from build123d import *

# Parameters (mm, degrees)
SKETCH1_W                  = 105
SKETCH1_H                  = 100
SKETCH1_W_2                = 4
SKETCH1_H_2                = 11
MAIN_PCB_DEPTH             = 1.25
MAIN_PCB_ROUNDED_CORNERS_R = 5
MAIN_PCB_HOLES_REACH       = 3.25
SKETCH2_R                  = 2
SKETCH2_R_2                = 1.375


with BuildPart() as part:
    # Sketch1 → Main PCB (new body)
    with BuildSketch(Plane(origin=(0, 0, 0), x_dir=(1, 0, 0), z_dir=(0, 1, 0))):
        Rectangle(SKETCH1_W, SKETCH1_H)
        with Locations((54.5, 19)):
            Rectangle(SKETCH1_W_2, SKETCH1_H_2)
    extrude(amount=MAIN_PCB_DEPTH)

    # Main PCB rounded corners
    main_pcb_rounded_corners_edges = [part.edges().sort_by_distance(p)[0] for p in [
        (52.5, 0.625, 50),
        (-52.5, 0.625, 50),
        (-52.5, 0.625, -50),
        (52.5, 0.625, -50),
    ]]
    fillet(main_pcb_rounded_corners_edges, radius=MAIN_PCB_ROUNDED_CORNERS_R)

    # Sketch2 → Main PCB holes (cut, up to next)
    with BuildSketch(Plane(origin=(0, 1.25, 0), x_dir=(1, 0, 0), z_dir=(0, 1, 0)), mode=Mode.PRIVATE) as main_pcb_holes_sk1:
        with Locations((-46.9, 46.65)):
            Circle(SKETCH2_R)
    main_pcb_holes_tool1 = extrude(main_pcb_holes_sk1.sketch, amount=-MAIN_PCB_HOLES_REACH, mode=Mode.PRIVATE) & part.part
    add(main_pcb_holes_tool1.solids().sort_by_distance((-46.9, 1.25, -46.65))[0], mode=Mode.SUBTRACT)
    # Sketch2 → Main PCB holes (cut, up to next)
    with BuildSketch(Plane(origin=(0, 1.25, 0), x_dir=(1, 0, 0), z_dir=(0, 1, 0)), mode=Mode.PRIVATE) as main_pcb_holes_sk2:
        with Locations((46.9, 46.65)):
            Circle(SKETCH2_R)
    main_pcb_holes_tool2 = extrude(main_pcb_holes_sk2.sketch, amount=-MAIN_PCB_HOLES_REACH, mode=Mode.PRIVATE) & part.part
    add(main_pcb_holes_tool2.solids().sort_by_distance((46.9, 1.25, -46.65))[0], mode=Mode.SUBTRACT)
    # Sketch2 → Main PCB holes (cut, up to next)
    with BuildSketch(Plane(origin=(0, 1.25, 0), x_dir=(1, 0, 0), z_dir=(0, 1, 0)), mode=Mode.PRIVATE) as main_pcb_holes_sk3:
        with Locations((46.9, -46.65)):
            Circle(SKETCH2_R)
    main_pcb_holes_tool3 = extrude(main_pcb_holes_sk3.sketch, amount=-MAIN_PCB_HOLES_REACH, mode=Mode.PRIVATE) & part.part
    add(main_pcb_holes_tool3.solids().sort_by_distance((46.9, 1.25, 46.65))[0], mode=Mode.SUBTRACT)
    # Sketch2 → Main PCB holes (cut, up to next)
    with BuildSketch(Plane(origin=(0, 1.25, 0), x_dir=(1, 0, 0), z_dir=(0, 1, 0)), mode=Mode.PRIVATE) as main_pcb_holes_sk4:
        with Locations((-46.9, -46.65)):
            Circle(SKETCH2_R)
    main_pcb_holes_tool4 = extrude(main_pcb_holes_sk4.sketch, amount=-MAIN_PCB_HOLES_REACH, mode=Mode.PRIVATE) & part.part
    add(main_pcb_holes_tool4.solids().sort_by_distance((-46.9, 1.25, 46.65))[0], mode=Mode.SUBTRACT)
    # Sketch2 → Main PCB holes (cut, up to next)
    with BuildSketch(Plane(origin=(0, 1.25, 0), x_dir=(1, 0, 0), z_dir=(0, 1, 0)), mode=Mode.PRIVATE) as main_pcb_holes_sk5:
        with Locations((-36.75, -48.625)):
            Circle(SKETCH2_R_2)
    main_pcb_holes_tool5 = extrude(main_pcb_holes_sk5.sketch, amount=-MAIN_PCB_HOLES_REACH, mode=Mode.PRIVATE) & part.part
    add(main_pcb_holes_tool5.solids().sort_by_distance((-36.75, 1.25, 48.625))[0], mode=Mode.SUBTRACT)
    # Sketch2 → Main PCB holes (cut, up to next)
    with BuildSketch(Plane(origin=(0, 1.25, 0), x_dir=(1, 0, 0), z_dir=(0, 1, 0)), mode=Mode.PRIVATE) as main_pcb_holes_sk6:
        with BuildLine():
            ThreePointArc((-36.75, -50), (-37.722271824, -49.597271824), (-38.125, -48.625))
            Line((-38.125, -48.625), (-38.125, -50))
            Line((-38.125, -50), (-36.75, -50))
        make_face()
    main_pcb_holes_tool6 = extrude(main_pcb_holes_sk6.sketch, amount=-MAIN_PCB_HOLES_REACH, mode=Mode.PRIVATE) & part.part
    add(main_pcb_holes_tool6.solids().sort_by_distance((-37.817869, 1.25, 49.692869))[0], mode=Mode.SUBTRACT)
    # Sketch2 → Main PCB holes (cut, up to next)
    with BuildSketch(Plane(origin=(0, 1.25, 0), x_dir=(1, 0, 0), z_dir=(0, 1, 0)), mode=Mode.PRIVATE) as main_pcb_holes_sk7:
        with BuildLine():
            Line((-35.375, -50), (-35.375, -48.625))
            ThreePointArc((-35.375, -48.625), (-35.777728176, -49.597271824), (-36.75, -50))
            Line((-36.75, -50), (-35.375, -50))
        make_face()
    main_pcb_holes_tool7 = extrude(main_pcb_holes_sk7.sketch, amount=-MAIN_PCB_HOLES_REACH, mode=Mode.PRIVATE) & part.part
    add(main_pcb_holes_tool7.solids().sort_by_distance((-35.682131, 1.25, 49.692869))[0], mode=Mode.SUBTRACT)
    # Sketch2 → Main PCB holes (cut, up to next)
    with BuildSketch(Plane(origin=(0, 1.25, 0), x_dir=(1, 0, 0), z_dir=(0, 1, 0)), mode=Mode.PRIVATE) as main_pcb_holes_sk8:
        with BuildLine():
            Line((-36.75, 50), (-38.125, 50))
            Line((-38.125, 50), (-38.125, 48.625))
            ThreePointArc((-38.125, 48.625), (-37.722271824, 49.597271824), (-36.75, 50))
        make_face()
    main_pcb_holes_tool8 = extrude(main_pcb_holes_sk8.sketch, amount=-MAIN_PCB_HOLES_REACH, mode=Mode.PRIVATE) & part.part
    add(main_pcb_holes_tool8.solids().sort_by_distance((-37.817869, 1.25, -49.692869))[0], mode=Mode.SUBTRACT)
    # Sketch2 → Main PCB holes (cut, up to next)
    with BuildSketch(Plane(origin=(0, 1.25, 0), x_dir=(1, 0, 0), z_dir=(0, 1, 0)), mode=Mode.PRIVATE) as main_pcb_holes_sk9:
        with Locations((-36.75, 48.625)):
            Circle(SKETCH2_R_2)
    main_pcb_holes_tool9 = extrude(main_pcb_holes_sk9.sketch, amount=-MAIN_PCB_HOLES_REACH, mode=Mode.PRIVATE) & part.part
    add(main_pcb_holes_tool9.solids().sort_by_distance((-36.75, 1.25, -48.625))[0], mode=Mode.SUBTRACT)
    # Sketch2 → Main PCB holes (cut, up to next)
    with BuildSketch(Plane(origin=(0, 1.25, 0), x_dir=(1, 0, 0), z_dir=(0, 1, 0)), mode=Mode.PRIVATE) as main_pcb_holes_sk10:
        with BuildLine():
            Line((-35.375, 50), (-36.75, 50))
            ThreePointArc((-36.75, 50), (-35.777728176, 49.597271824), (-35.375, 48.625))
            Line((-35.375, 48.625), (-35.375, 50))
        make_face()
    main_pcb_holes_tool10 = extrude(main_pcb_holes_sk10.sketch, amount=-MAIN_PCB_HOLES_REACH, mode=Mode.PRIVATE) & part.part
    add(main_pcb_holes_tool10.solids().sort_by_distance((-35.682131, 1.25, -49.692869))[0], mode=Mode.SUBTRACT)


solid = part.part
Model file for the job. Use its own axes, mm. Give positions to 0.01 mm unless a question says otherwise; leave off trailing zeros. Order: outer loops, then holes, each group sorted by start corner. A loop starts at its lowest first (then second) coordinate and runs counter-clockwise, first axis right, second up. Notation, with made-up numbers: (-27, -32.75) - (-19, -32.75) arc R25 cw to (-19, -6.75) - close; hole circle Ø3 at (38, 34). An arc over 180 degrees is marked (long way). One line per item, written item: value.
Item 1: Two-plate mould, pull along Z, no slides. Class faces 1 (the cylindrical face through (46.466, 0.634, 48.602)), 2 (the cylindrical face through (51, 0.63, 48.57)), 3 (the flat face through (1, 0, -1)): released by +Z, released by -Z, zero draft, split by the parting line, or undercut.
Response values:
face 1: undercut
face 2: released by +Z
face 3: zero draft
Item 2: Slice it at C-C (x = -36.75). List the corners of the cut face in (y, z).
Response values:
outline: (0, -47.25) - (1.25, -47.25) - (1.25, 47.25) - (0, 47.25) - close
Item 3: Slice it at A-A (y = 0.85). List the corners of the cut face in (x, z) (3 decimals).
Response values:
outline: (-52.5, -45) arc R5 ccw to (-47.5, -50) - (-38.125, -50) - (-38.125, -48.625) arc R1.375 cw to (-35.375, -48.625) - (-35.375, -50) - (47.5, -50) arc R5 ccw to (52.5, -45) - (52.5, -24.5) - (56.5, -24.5) - (56.5, -13.5) - (52.5, -13.5) - (52.5, 45) arc R5 ccw to (47.5, 50) - (-35.375, 50) - (-35.375, 48.625) arc R1.375 cw to (-38.125, 48.625) - (-38.125, 50) - (-47.5, 50) arc R5 ccw to (-52.5, 45) - close; hole circle Ø4 at (-46.9, -46.65); hole circle Ø4 at (-46.9, 46.65); hole circle Ø4 at (46.9, -46.65); hole circle Ø4 at (46.9, 46.65)
Item 4: Pin check, flat tips, straight feed: pin 1 Ø3 at (x, z) = (-46.9, -46.65) entering from +Y; pin 2 Ø0.6 at (y, z) = (0.5, 49.5) entering from +X. Stop position of each tip, or through.
Response values:
pin 1: through
pin 2: x = 50.21
Item 5: Slice it at B-B (z = 43). List the corners of the cut face in (x, y), then the cut area to 3 significant figures.
Response values:
outline: (-52.5, 0) - (52.5, 0) - (52.5, 1.25) - (-52.5, 1.25) - close
area: 131 mm2
Item 6: Wall check: line 1 (Z direction, x = -46.9, y = 0.45); line 2 (X direction, y = 0.35, z = -46.65); line 3 (X direction, y = 0.4, z = 34.5). Give the ranges that are in metal, low to high.
Response values:
line 1: -50 to -48.65, -44.65 to 44.65, 48.65 to 50
line 2: -52.22 to -48.9, -44.9 to 44.9, 48.9 to 52.22
line 3: -52.5 to 52.5
